The listing builds one solid part. Answer for the finished solid, in the listing's coordinates (mm). A direction names the side the tool comes from. Give positions to 0.01 mm unless a question says otherwise; leave off trailing zeros. Order: outer loops, then holes, each group sorted by start corner. A loop starts at its lowest first (then second) coordinate and runs counter-clockwise, first axis right, second up. Notation, with made-up numbers: (29.25, 55) - (38.25, 55) arc R24 cw to (38.25, 78) - close; hole circle Ø11 at (3, -39). An arc over 180 degrees is marked (long way). Use a Markdown table: item, result. Add a question column.
1) Find section C-C, the plane z = 2.5. Determine the outline of the cut face in (x, y) (3 decimals).
2) Straight lines are drawn through the part: line 1 (X direction, y = -12.5, z = 2.5); line 2 (Y direction, x = 589.5, z = 6.5); line 3 (Z direction, x = 605, y = -1.5). For each, find the intervals that lie inside material, in ascending order.
3) Flat-ended cylindrical pins translate along their axes: pin 1 (12 mm diameter, centred on x = 560, y = -23, fed in from +Z); pin 2 (2 mm diameter, centred on x = 583.5, y = -4.5, fed in from +Z). Find the tip coordinate at first contact, or state that the pin passes through.
4) Find section B-B, the plane x = 536. Determine the outline of the cut face in (y, z).
5) Find section A-A, the plane y = -18. Determine the outline of the cut face in (x, z).
6) For faces 4 (the face through (565, -26, 0)), 5 (the face through (528, -24.49, 3.56)), determine the directions among +Z, -Z, +X, -X, +Y, -Y from which every point of the face is accessible in a straight line to the end or side of a thin tool.
7) The mould has two halves that part along X. Classify faces 1 (the face through (520.7, -16, 4)), 2 (the face through (602.34, -24.45, 3.88)), 3 (the face through (565, -31.75, 4)): released by +X, released by -X, zero draft, split by the parting line, or undercut.
from build123d import *

# Parameters (mm, degrees)
F3_DEPTH = 31.75
F5_DEPTH = 7.9385
F6_R     = 5.08


with BuildPart() as f3:
    # F1 (on Front) → F3 (new body)
    with BuildSketch(Plane.XZ):
        Polygon((609.6, 0), (609.6, 7.9375), (520.7, 7.127214), (520.7, 0), align=None)
    extrude(amount=F3_DEPTH)

    # F4 (on face) → F5 (cut, through all)
    with BuildSketch(Plane(origin=(0, 0, 0), x_dir=(1, 0, 0), z_dir=(0, 0, -1))):
        with BuildLine():
            Line((600.075, 25.4), (530.225, 25.4))
            ThreePointArc((530.225, 25.4), (527.979936, 24.470064), (527.05, 22.225))
            Line((527.05, 22.225), (527.05, 9.525))
            ThreePointArc((527.05, 9.525), (527.979936, 7.279936), (530.225, 6.35))
            Line((530.225, 6.35), (600.075, 6.35))
            ThreePointArc((600.075, 6.35), (602.320064, 7.279936), (603.25, 9.525))
            Line((603.25, 9.525), (603.25, 22.225))
            ThreePointArc((603.25, 22.225), (602.320064, 24.470064), (600.075, 25.4))
        make_face()
    extrude(amount=-F5_DEPTH, mode=Mode.SUBTRACT)

    # F6
    f6_edges = [f3.edges().sort_by_distance(p)[0] for p in [
        (520.7, -31.75, 3.563607),
        (520.7, 0, 3.563607),
        (609.6, -31.75, 3.96875),
        (609.6, 0, 3.96875),
    ]]
    fillet(f6_edges, radius=F6_R)


solid = f3.part
The answers:
| question | item | result |
|---|---|---|
| 1 | outline | (520.7, -26.67) arc R5.08 ccw to (525.78, -31.75) - (604.52, -31.75) arc R5.08 ccw to (609.6, -26.67) - (609.6, -5.08) arc R5.08 ccw to (604.52, 0) - (525.78, 0) arc R5.08 ccw to (520.7, -5.08) - close; hole (527.05, -22.225) arc R3.175 ccw to (530.225, -25.4) - (600.075, -25.4) arc R3.175 ccw to (603.25, -22.225) - (603.25, -9.525) arc R3.175 ccw to (600.075, -6.35) - (530.225, -6.35) arc R3.175 ccw to (527.05, -9.525) - close |
| 2 | line 1 | 520.7 to 527.05, 603.25 to 609.6 |
| 2 | line 2 | -31.75 to -25.4, -6.35 to 0 |
| 2 | line 3 | 0 to 7.9 |
| 3 | pin 1 | z = 7.54 |
| 3 | pin 2 | z = 7.71 |
| 4 | outline | (-31.75, 0) - (-25.4, 0) - (-25.4, 7.27) - (-31.75, 7.27) - close; (-6.35, 0) - (0, 0) - (0, 7.27) - (-6.35, 7.27) - close |
| 5 | outline | (520.7, 0) - (527.05, 0) - (527.05, 7.19) - (520.7, 7.13) - close; (603.25, 0) - (609.6, 0) - (609.6, 7.94) - (603.25, 7.88) - close |
| 6 | face 4 | -Z, +X, -X, +Y, -Y |
| 6 | face 5 | +Z, -Z |
| 7 | face 1 | released by -X |
| 7 | face 2 | undercut |
| 7 | face 3 | zero draft |
